Could you check a few things on this model? Use its own coordinates, in mm. A direction names the side the tool comes from. Round coordinates to 2 decimals unless told otherwise and drop trailing zeros. Loops run counter-clockwise (first coordinate to the right, second up) from the corner with the lowest first, then second, coordinate; pieces in that order, holes last. Notation, with made-up numbers: (84, 13) -> (136, 13) arc R22 ccw to (136, 38) -> close; hole circle Ø3 at (-3, 20). An arc over 180 degrees is marked (long way). Write each question's results on one line, items separated by ' | '.
from build123d import *

# Parameters (mm, degrees)
BOSS_EXTRU_1_DEPTH      = 2.5
BOSS_EXTRU_1_DEPTH_BACK = 2.5
ESQUISSE2_R             = 0.5


with BuildPart() as part:
    # Esquisse1 → Révolution1 (revolve)
    with BuildSketch(Plane(origin=(0, 0, 0), x_dir=(0, 0, -1), z_dir=(1, 0, 0))):
        with BuildLine():
            Line((1.49716245, 12.907779617), (1.5, 13))
            ThreePointArc((1.5, 13), (1.060660172, 14.060660172), (0, 14.5))
            Line((0, 14.5), (0, -0.857830241))
            Line((0, -0.857830241), (1.1, -0.857830241))
            Line((1.1, -0.857830241), (1.1, 0))
            Line((1.1, 0), (1.49716245, 12.907779617))
        make_face()
    revolve(axis=Axis((0, 0, 0), (0, 1, 0)))

    # Esquisse2 → Boss.-Extru.1 (add, two sides: drawn at the far end of the back side and taken through both)
    with BuildSketch(Plane(origin=(0, 0, 0), x_dir=(0, 0, -1), z_dir=(1, 0, 0)).offset(-BOSS_EXTRU_1_DEPTH_BACK)):
        Circle(ESQUISSE2_R)
    extrude(amount=BOSS_EXTRU_1_DEPTH + BOSS_EXTRU_1_DEPTH_BACK)


solid = part.part
1) I want a section at B-B, the plane y = 4. Write out the boundary of the cut face in (x, z), plus the area to 3 significant figures.
Model answer:
outline: circle Ø2.45 at (0, 0) | area: 4.70 mm2
2) I need wall thicknesses on line 1 (Y direction, x = 0.6, z = 0.2); line 2 (X direction, y = 12.5, z = -0.8); line 3 (Z direction, x = -0.5, y = 0). Which ranges of each line are inside material? Lowest first, please.
Model answer:
line 1: y = -0.86 to 14.36 | line 2: x = -1.25 to 1.25 | line 3: z = -0.98 to 0.98
3) I want a section at A-A, the plane y = 6.5. Write out the boundary of the cut face in (x, z).
Model answer:
outline: circle Ø2.6 at (0, 0)
4) For faces 1 (the cylindrical face through (-0.33, -0.42, -1.05)), 2 (the cylindrical face through (1.7, 0, 0.5)), 3 (the cylindrical face through (-1.8, 0, 0.5)), which set-ups out of +Z, -Z, +X, -X, +Y, -Y let a thin tool reach every point of the face, with its end or its side?
Model answer:
face 1: -Y | face 2: +X | face 3: -X
5) I'm going to push flat-ended pins straight in: pin 1 (1.5 mm diameter, centred on x = 1.5, z = 1, fed in from +Y); pin 2 (1.5 mm diameter, centred on y = 9, z = 0, fed in from +X). Where does each tip first touch, or does it pass through?
Model answer:
pin 1: stops at y = 14.07 | pin 2: stops at x = 1.4
